Source: CAD feature listing. Evaluate the final solid. Frame: model axes, mm. Face numbers are marked on the shaded views. A direction names the side the tool comes from. Round coordinates to 2 decimals unless told otherwise and drop trailing zeros. Loops run counter-clockwise (first coordinate to the right, second up) from the corner with the lowest first, then second, coordinate; pieces in that order, holes last. Notation, with made-up numbers: M 33.25,-21 L 69.25,-21 A29 cw 69.25,14 Z; hole C -34.5,60.5 d4. An arc over 180 degrees is marked long. One line per item, written item: value.
from build123d import *

# Parameters (mm, degrees)
SKETCH017_R             = 4
PAD005_DEPTH            = 12
PAD006_DEPTH            = 21
SKETCH020_R             = 11.9
PAD007_DEPTH            = 1
BODY004_PLACEMENT_ANGLE = 180


with BuildPart() as part:
    # Sketch017 → Pad005 (new body)
    with BuildSketch(Plane.YZ):
        Circle(SKETCH017_R)
    extrude(amount=PAD005_DEPTH)

    # Sketch018 → Pad006 (join)
    with BuildSketch(Plane.YZ):
        with BuildLine():
            ThreePointArc((1.9, 1.296148), (-2.3, 0), (1.9, -1.296148))
            Line((1.9, -0.65), (1.9, -1.296148))
            Line((1.4, -0.65), (1.9, -0.65))
            Line((1.4, 0.65), (1.4, -0.65))
            Line((1.9, 0.65), (1.4, 0.65))
            Line((1.9, 1.296148), (1.9, 0.65))
        make_face()
    extrude(amount=-PAD006_DEPTH)

    # Sketch020 (on Face3 of Pad006) → Pad007 (join)
    with BuildSketch(Plane.YZ.offset(12)):
        Circle(SKETCH020_R)
    extrude(amount=-PAD007_DEPTH)


with BuildPart() as part_1:
    # Body004 placement: moved
    add(part.part.moved(Location((-22, 0, 0))).rotate(Axis((-22, 0, 0), (0, 1, 0)), BODY004_PLACEMENT_ANGLE))


solid = part_1.part
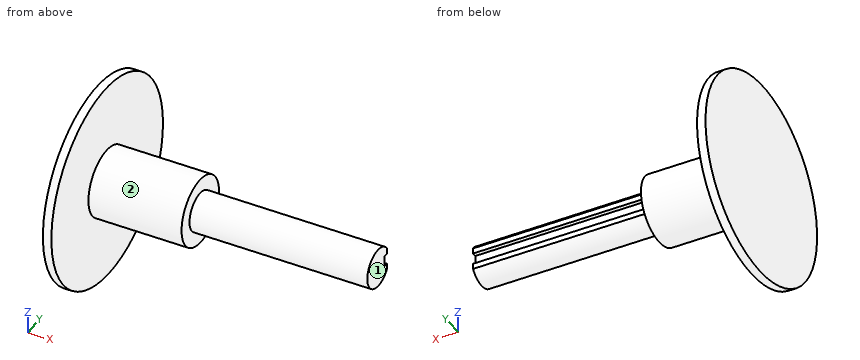
1. Section query A-A (y = 0). Return the cut outline in (x, z).
Report:
outline: M -34,-11.9 L -33,-11.9 L -33,-4 L -22,-4 L -22,-2.3 L -1,-2.3 L -1,2.3 L -22,2.3 L -22,4 L -33,4 L -33,11.9 L -34,11.9 Z
2. Section query D-D (x = -23). Return the cut outline in (y, z).
Report:
outline: C 0,0 d8
3. Reachability of the marked faces 1 and 2 from +Z, -Z, +X, -X, +Y, -Y: full face, straight path, thin tool, end or side. Return the list, or none.
Report:
face 1: +Z, -Z, +X, +Y, -Y
face 2: +X
4. Ray query, line 1 (X direction, y = 6.5, z = -0.5); line 2 (X direction, y = -2.75, z = 1.5); line 3 (Z direction, x = -4, y = -2). Return the intervals inside material, ascending. Write a range as [from, to].
Report:
line 1: x = [-34, -33]
line 2: x = [-34, -22]
line 3: z = [-1.14, 1.14]
5. Section query C-C (x = -11). Return the cut outline in (y, z), and give its area (3 significant figures).
Report:
outline: M 1.4,-0.65 L 1.4,0.65 L 1.9,0.65 L 1.9,1.3 A2.3 ccw long 1.9,-1.3 L 1.9,-0.65 Z
area: 15.3 mm2
6. Pin query (flat end, axial travel): pin 1 (8 mm diameter, centred on x = -5, y = -0.5, fed in from +Z); pin 2 (0.7 mm diameter, centred on x = -15.5, z = 1, fed in from +Y); pin 3 (2 mm diameter, centred on x = -29.5, z = 1.5, fed in from +Y). Return the tip coordinate at first contact, or that it passes through.
Report:
pin 1: stops at z = 2.3
pin 2: stops at y = 1.9
pin 3: stops at y = 3.97
7. Section query B-B (z = 0). Return the cut outline in (x, y), and give its area (4 significant figures).
Report:
outline: M -34,-11.9 L -33,-11.9 L -33,-4 L -22,-4 L -22,-2.3 L -1,-2.3 L -1,1.4 L -22,1.4 L -22,4 L -33,4 L -33,11.9 L -34,11.9 Z
area: 189.5 mm2
